The model under review builds one solid part; all positions refer to its coordinate system, in mm. A direction names the side the tool comes from. Round coordinates to 2 decimals unless told otherwise and drop trailing zeros. Order: outer loops, then holes, each group sorted by start corner. A loop starts at its lowest first (then second) coordinate and runs counter-clockwise, first axis right, second up.
1) Consider section A-A (z = 12). Give the boundary of the cut face in (x, y), then the cut area to 3 significant figures.
2) Mouldability with a two-part tool opening along Y and no side actions: class faces 1 (the face through (62.001, -38, 38)), 2 (the face through (-63.5, -1, 38)), 3 (the face through (-1, 76.2, 38)), 4 (the face through (-52.61, -63.758, 33.297)) as pulls with the +Y half, pulls with the -Y half, needs draft (parallel to the pull), parting line crosses it, or undercut.
3) Consider section C-C (y = 36). Give the boundary of the cut face in (x, z), then the cut area to 3 significant figures.
4) Machinability: for faces 5 (the face through (-41.453, -38, 38)), 6 (the face through (-19, 0, 76.2)), which of the approach directions +Z, -Z, +X, -X, +Y, -Y give a long, thin tool a straight path to every point of the face, cutting with its end or side? Answer none if there is none.
5) To check wall thickness, follow L1, parallel to Y at x = 22.5, z = 62; L2, parallel to X at y = 26, z = 70; L3, parallel to X at y = -23.5, z = 39. State the ranges of each line that lie inside material, in increasing order.
6) Clearance check with flat-ended pins moving along their axes: P1, Ø1.2, axis at x = -52.5, y = -75.5, coming from the +Z side; P2, Ø5.5, axis at x = -57, z = 47.5, coming from the -Y side; P3, Ø4, axis at x = -49, y = 43, coming from the +Z side. State where each tip first meets the part, or that it passes through.
7) Consider section B-B (z = 45.5). Give the boundary of the cut face in (x, y), then the cut area to 3 significant figures.
8) Consider section D-D (x = -5.5). Give the boundary of the cut face in (y, z).
from build123d import *

# Parameters (mm, degrees)
F0_W      = 127
F0_H      = 152.4
F1_DEPTH  = 76.2
F2_T      = -1.4986
F3_W      = 1.4986
F3_H      = 149.4028
F4_DEPTH  = 74.7014
F5_W      = 103.4542
F5_H      = 1.4986
F6_DEPTH  = 74.7014
F8_DEPTH  = 20.5486
F9_W      = 19.05
F9_H      = 38.6785856472
F10_DEPTH = 4.064


# Not quite as in the source:
# - an extrude ends at something that could not be found from the text; its depth is read off the source's solid


with BuildPart() as f1:
    # F0 (on Top) → F1 (new body)
    with BuildSketch(Plane.XY):
        Rectangle(F0_W, F0_H)
    extrude(amount=F1_DEPTH)

    # F2
    f2_openings = [f1.faces().sort_by_distance(p)[0] for p in [
        (0, 0, 76.2),
    ]]
    offset(amount=F2_T, openings=f2_openings)

    # F3 (on face) → F4 (join, through all)
    with BuildSketch(Plane.XY.offset(1.4986)):
        with Locations((-42.2021, 0)):
            Rectangle(F3_W, F3_H)
    extrude(amount=F4_DEPTH)

    # F5 (on face) → F6 (join, through all)
    with BuildSketch(Plane.XY.offset(1.4986)):
        with Locations((10.2743, 0)):
            Rectangle(F5_W, F5_H)
    extrude(amount=F6_DEPTH)

    # F7 (on face) → F8 (join, through all)
    with BuildSketch(Plane(origin=(-63.5, 0, 0), x_dir=(0, -1, 0), z_dir=(-1, 0, 0))):
        Polygon((76.2, 0), (76.2, 38.1), (52.5047014133, 28.9516217345), (36.4950394487, 70.4183942612), (-76.2, 26.9086302568), (-76.2, 0), align=None)
    extrude(amount=-F8_DEPTH)

    # F9 (on face) → F10 (cut)
    with BuildSketch(Plane(origin=(0, -74.7014, 0), x_dir=(-1, 0, 0), z_dir=(0, 1, 0))):
        with Locations((52.4764, 56.8607071764)):
            Rectangle(F9_W, F9_H)
    extrude(amount=-F10_DEPTH, mode=Mode.SUBTRACT)


solid = f1.part
Answer below:
1. outline: (-63.5, -76.2) - (63.5, -76.2) - (63.5, 76.2) - (-63.5, 76.2) - close; hole (-41.45, -74.7) - (62, -74.7) - (62, -0.75) - (-41.45, -0.75) - close; hole (-41.45, 0.75) - (62, 0.75) - (62, 74.7) - (-41.45, 74.7) - close
1. area: 4,050 mm2
2. face 1: undercut
2. face 2: needs draft
2. face 3: pulls with the +Y half
2. face 4: undercut
3. outline: (-63.5, 0) - (63.5, 0) - (63.5, 76.2) - (62, 76.2) - (62, 1.5) - (-41.45, 1.5) - (-41.45, 76.2) - (-42.95, 76.2) - (-42.95, 42.43) - (-62, 42.43) - (-62, 76.2) - (-63.5, 76.2) - close
3. area: 1,310 mm2
4. face 5: +Z
4. face 6: +Z, +X, -X, +Y, -Y
5. L1: y = -76.2 to -74.7, -0.75 to 0.75, 74.7 to 76.2
5. L2: x = -63.5 to -62, -42.95 to -41.45, 62 to 63.5
5. L3: x = -63.5 to -41.45, 62 to 63.5
6. P1: stops at z = 37.52
6. P2: stops at y = -46.41
6. P3: stops at z = 40.5
7. outline: (-63.5, -76.2) - (-62, -76.2) - (-62, -46.12) - (-42.95, -46.12) - (-42.95, -76.2) - (63.5, -76.2) - (63.5, 76.2) - (-63.5, 76.2) - close; hole (-62, 28.05) - (-42.95, 28.05) - (-42.95, 74.7) - (-62, 74.7) - close; hole (-41.45, -74.7) - (62, -74.7) - (62, -0.75) - (-41.45, -0.75) - close; hole (-41.45, 0.75) - (62, 0.75) - (62, 74.7) - (-41.45, 74.7) - close
7. area: 2,590 mm2
8. outline: (-76.2, 0) - (76.2, 0) - (76.2, 76.2) - (74.7, 76.2) - (74.7, 1.5) - (0.75, 1.5) - (0.75, 76.2) - (-0.75, 76.2) - (-0.75, 1.5) - (-74.7, 1.5) - (-74.7, 76.2) - (-76.2, 76.2) - close
